```python
from build123d import *

# Parameters (mm, degrees)
SKETCH1_W               = 8
SKETCH1_H               = 8
BOSS_EXTRUDE1_DEPTH     = 3
CUT_EXTRUDE1_DEPTH      = 12.704699911
CUT_EXTRUDE1_DEPTH_BACK = 12.704699911
CUT_EXTRUDE2_DEPTH      = 11
SKETCH4_R               = 1.8
CUT_EXTRUDE3_DEPTH      = 0.8
SKETCH5_W               = 8
SKETCH5_H               = 1
BOSS_EXTRUDE2_DEPTH     = 2
FILLET1_R               = 4
CUT_EXTRUDE4_DEPTH      = 0.4


with BuildPart() as part:
    # Sketch1 → Boss-Extrude1 (new body)
    with BuildSketch(Plane(origin=(0, 0, 0), x_dir=(1, 0, 0), z_dir=(0, 1, 0))):
        with Locations((4, 4)):
            Rectangle(SKETCH1_W, SKETCH1_H)
    extrude(amount=BOSS_EXTRUDE1_DEPTH)

    # Sketch2 → Cut-Extrude1 (cut, two sides: drawn at the far end of the back side and taken through both)
    with BuildSketch(Plane.XY.offset(-CUT_EXTRUDE1_DEPTH_BACK)):
        Polygon((0, 0), (0.6, 3), (0, 3), align=None)
        Polygon((8, 0), (7.4, 3), (8, 3), align=None)
    extrude(amount=CUT_EXTRUDE1_DEPTH + CUT_EXTRUDE1_DEPTH_BACK, mode=Mode.SUBTRACT)

    # Sketch3 → Cut-Extrude2 (cut)
    with BuildSketch(Plane(origin=(0, 0, 0), x_dir=(0, 0, -1), z_dir=(1, 0, 0))):
        Polygon((0, 0), (0.6, 3), (0, 3), align=None)
        Polygon((8, 3), (7.4, 3), (8, 0), align=None)
    extrude(amount=CUT_EXTRUDE2_DEPTH, mode=Mode.SUBTRACT)

    # Sketch4 → Cut-Extrude3 (cut)
    with BuildSketch(Plane.XZ):
        with Locations(Location((4, -3.75, 0), (0, 0, 270))):
            Circle(SKETCH4_R)
    extrude(amount=-CUT_EXTRUDE3_DEPTH, mode=Mode.SUBTRACT)

    # Sketch5 → Boss-Extrude2 (add)
    with BuildSketch(Plane.XZ):
        with Locations((4, -7.5)):
            Rectangle(SKETCH5_W, SKETCH5_H)
    extrude(amount=BOSS_EXTRUDE2_DEPTH)

    # Fillet1
    # the kernel refuses this fillet: 4 mm, written as the material it takes off along each edge
    with BuildSketch(Plane(origin=(8, -2, -16.660254038), x_dir=(0, 1, 0), z_dir=(0, 0, 1)), Plane(origin=(0, -2, 1.660254038), x_dir=(0, 1, 0), z_dir=(0, 0, -1))) as fillet1_piece_1:
        with BuildLine():
            CenterArc((4, 3.464101615), FILLET1_R, 180, 60)
            Line((0, 3.464101615), (-0.08, 3.464101615))
            Line((-0.08, 3.464101615), (-0.08, 0))
            Line((-0.08, 0), (0, -0.08))
            ThreePointArc((0, -0.08), (1, -0.08), (1.96, -0.069282032))
            Line((1.96, -0.069282032), (2, 0))
        make_face()
    extrude(amount=18.320508076, mode=Mode.SUBTRACT)

    # Sketch6 → Cut-Extrude4 (cut)
    with BuildSketch(Plane(origin=(0, 3, 0), x_dir=(1, 0, 0), z_dir=(0, 1, 0))):
        Polygon((3.039241423, 1.586469201), (4.258191744, 6.586469201), (4.982350398, 6.586469201), (3.76440168, 1.586469201), align=None)
    extrude(amount=-CUT_EXTRUDE4_DEPTH, mode=Mode.SUBTRACT)


solid = part.part
```
Source: CAD feature listing. Evaluate the final solid. Frame: model axes, mm. A direction names the side the tool comes from. Round coordinates to 2 decimals unless told otherwise and drop trailing zeros. Loops run counter-clockwise (first coordinate to the right, second up) from the corner with the lowest first, then second, coordinate; pieces in that order, holes last.
1. Contact query for a flat-ended pin moving along its axis: pin 1 (4 mm diameter, centred on x = 5, z = -3, fed in from -Y). Output: stop coordinate, or through.
2. Section query D-D on x = 1. Output: boundary loops of the cut face in (y, z).
3. Ray query, L1, parallel to Y at x = 6.5, z = -3; L2, parallel to Z at x = 3.5, y = -1.3; L3, parallel to X at y = 0.35, z = -3.75. Return the intervals inside material, ascending.
4. Mould query, pull axis X, two halves, no side actions, for faces 5 (the flat face through (3.9, 1.5, -0.3)), 6 (the flat face through (4, 0.8, -4)), 7 (the cylindrical face through (6.51, -1.48, -7.51)), 8 (the cylindrical face through (1.49, -1.48, -7.49)). Classes: released by +X, released by -X, zero draft, split by the parting line, or undercut.
5. Section query C-C on y = 1.35. Output: boundary loops of the cut face in (x, z).
6. Section query B-B on x = 4. Output: boundary loops of the cut face in (y, z).
7. Access query for faces 1 (the flat face through (4.38, 2.8, -4.12)), 2 (the flat face through (4, -1, -7)), 3 (the cylindrical face through (4.541, 0.394, -5.467)), 4 (the flat face through (3, 3, -4)). Directions: +Z, -Z, +X, -X, +Y, -Y. A direction counts if a zero-diameter tool reaches every point of the face in a straight line with its end or side. Return the directions, or none.
8. Section query A-A on z = -0.75. Output: boundary loops of the cut face in (x, y), and give its area (3 significant figures).
Answers below:
1. pin 1: stops at y = 0
2. outline: (-1.15, -8) - (0, -8) - (3, -7.4) - (3, -0.6) - (0, 0) - (0, -7) - (-1.15, -7) - close
3. L1: y = 0 to 3
3. L2: z = -8 to -7
3. L3: x = 0.07 to 2.2, 5.8 to 7.93
4. face 5: zero draft
4. face 6: undercut
4. face 7: released by +X
4. face 8: released by -X
5. outline: (0.27, -7.73) - (7.73, -7.73) - (7.73, -0.27) - (0.27, -0.27) - close
6. outline: (-2, -8) - (0, -8) - (3, -7.4) - (3, -5.53) - (2.6, -5.53) - (2.6, -2.55) - (3, -2.55) - (3, -0.6) - (0, 0) - (0, -1.95) - (0.8, -1.95) - (0.8, -5.55) - (0, -5.55) - (0, -7) - (-2, -7) - close
7. face 1: +Y
7. face 2: +Z, +X, -X, -Y
7. face 3: -Y
7. face 4: +Z, -Z, +X, -X, +Y
8. outline: (0, 0) - (8, 0) - (7.4, 3) - (0.6, 3) - close
8. area: 22.2 mm2
